Design review of the part shown in the three views and the two pictorial views. Dimensions are in mm from the part's minimum x, y and z. Coordinates: 2 decimals unless noted, no trailing zeros. Write each loop counter-clockwise with the first axis right and the second up, starting at its lowest first coordinate (ties: lowest second). Pieces come first, ordered by that corner, then holes. Notation, with made-up numbers: (62, 6.5) -> (106, 6.5) arc R24 cw to (106, 38.5) -> close; hole circle Ø9 at (4, 53). An arc over 180 degrees is marked (long way). Answer in a Markdown table with one row per item. Add a question column.
Item 1: Take a section at B-B, the plane x = 76.2. Write out the cut boundary in (y, z) (1 decimal), and give its area (3 significant figures).
Item 2: To check wall thickness, follow line 1 (X direction, y = 2.3, z = 203.2); line 2 (X direction, y = 2.5, z = 57.5); line 3 (Z direction, x = 61.5, y = 2.6) (1 decimal). State the ranges of each line that lie inside material, in increasing order.
Item 3: Take a section at A-A, the plane z = 127. Write out the cut boundary in (x, y) (1 decimal).
Item 4: Take a section at C-C, the plane y = 1.5. Give the number of separate pieces and of enclosed holes in the cut face, and give its area (3 significant figures).
Item 5: Clearance check with a flat-ended pin moving along its axis: P1, Ø4, axis at x = 93.98, z = 127, coming from the -Y side. State where the tip first meets the part, or that it passes through.
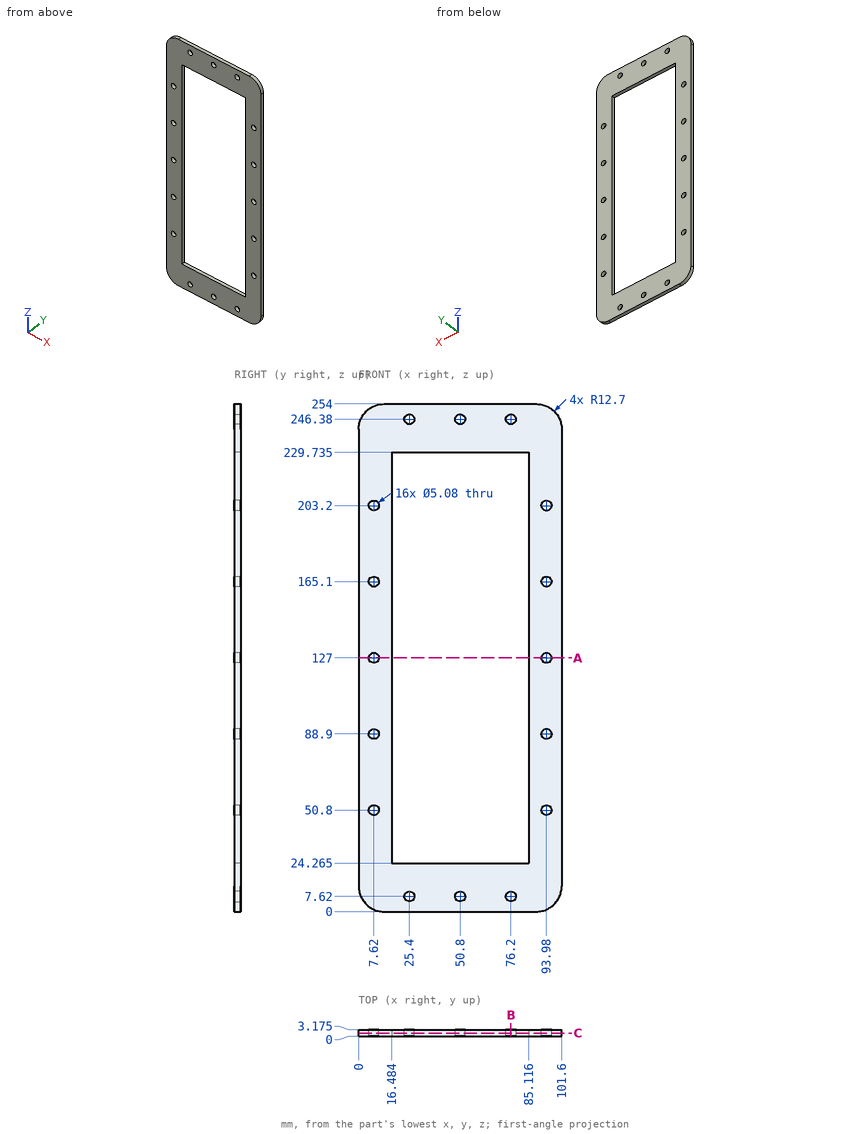
Answers:
| question | item | result |
|---|---|---|
| 1 | outline | (0, 0) -> (3.2, 0) -> (3.2, 5.1) -> (0, 5.1) -> close; (0, 10.2) -> (3.2, 10.2) -> (3.2, 24.3) -> (0, 24.3) -> close; (0, 229.7) -> (3.2, 229.7) -> (3.2, 243.8) -> (0, 243.8) -> close; (0, 248.9) -> (3.2, 248.9) -> (3.2, 254) -> (0, 254) -> close |
| 1 | area | 122 mm^2 |
| 2 | line 1 | x = 0 to 5.08, 10.16 to 16.48, 85.12 to 91.44, 96.52 to 101.6 |
| 2 | line 2 | x = 0 to 16.48, 85.12 to 101.6 |
| 2 | line 3 | z = 0 to 24.3, 229.7 to 254 |
| 3 | outline | (0, 0) -> (5.1, 0) -> (5.1, 3.2) -> (0, 3.2) -> close; (10.2, 0) -> (16.5, 0) -> (16.5, 3.2) -> (10.2, 3.2) -> close; (85.1, 0) -> (91.4, 0) -> (91.4, 3.2) -> (85.1, 3.2) -> close; (96.5, 0) -> (101.6, 0) -> (101.6, 3.2) -> (96.5, 3.2) -> close |
| 4 | separate pieces | 1 |
| 4 | enclosed holes | 17 |
| 4 | area | 11,200 mm^2 |
| 5 | P1 | passes through |
